Part print with two shaded views. Sizes in mm from the minimum x, y, z corner. Give positions to 0.01 mm unless a question says otherwise; leave off trailing zeros. Order: outer loops, then holes, each group sorted by start corner. A loop starts at its lowest first (then second) coordinate and runs counter-clockwise, first axis right, second up.
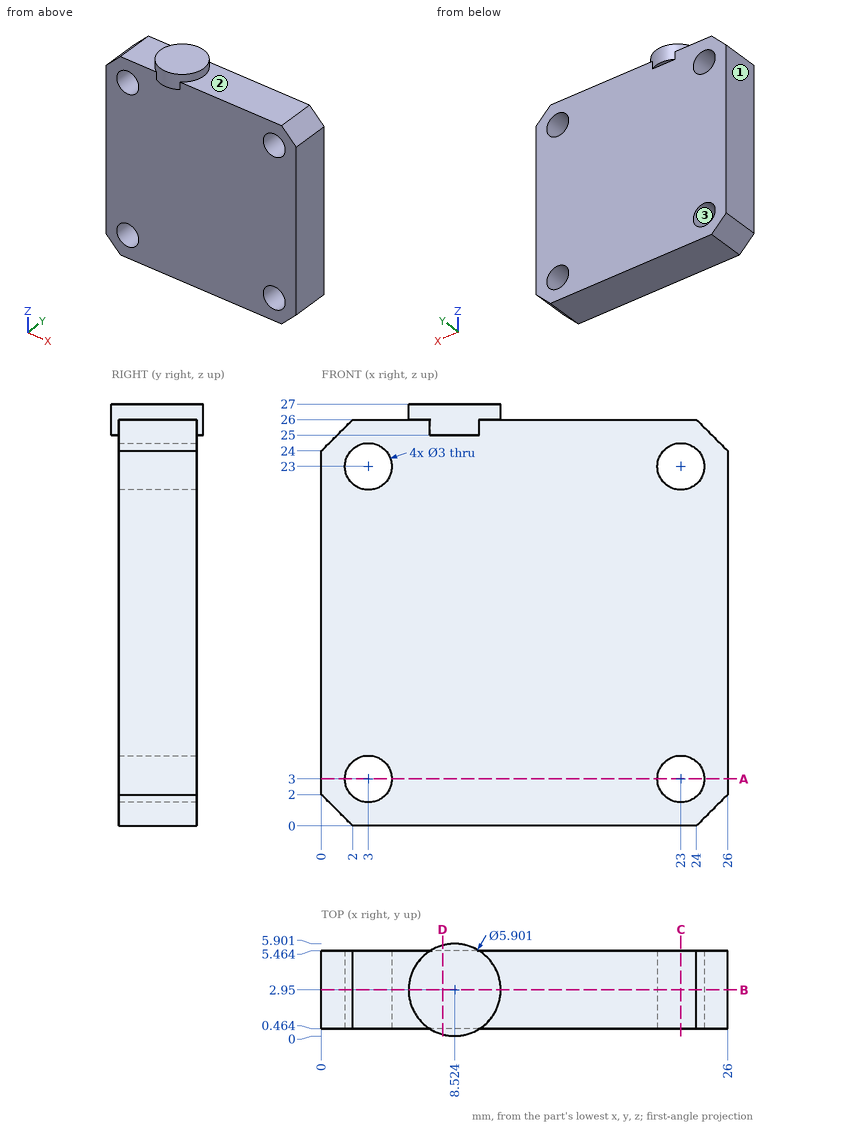
1. Saw through at D-D on x = 7.75. Give the cut face in (y, z), plus the area to 3 significant figures.
2. Saw through at C-C on x = 23. Give the cut face in (y, z).
3. Pin check, flat tips, straight feed: P1, Ø4, axis at x = 3, z = 23, coming from the +Y side; P2, Ø3.5, axis at x = 23, z = 3, coming from the -Y side. Stop position of each tip, or through.
4. Mould opens along Z. For the marked faces 1, 2 and 3 say: released by +Z, released by -Z, zero draft, split by the parting line, or undercut.
5. Saw through at A-A on z = 3. Give the cut face in (x, y).
6. Saw through at B-B on y = 2.95. Give the cut face in (x, z).
7. Wall check: line 1 (X direction, y = 2.4, z = 23); line 2 (X direction, y = 3.2, z = 2); line 3 (Z direction, x = 21.75, y = 4.5). Give the ranges that are in metal, low to high.
Reported:
1. outline: (0.1, 25) - (0.46, 25) - (0.46, 0) - (5.46, 0) - (5.46, 25) - (5.8, 25) - (5.8, 27) - (0.1, 27) - close
1. area: 136 mm2
2. outline: (0.46, 0) - (5.46, 0) - (5.46, 1.5) - (0.46, 1.5) - close; (0.46, 4.5) - (5.46, 4.5) - (5.46, 21.5) - (0.46, 21.5) - close; (0.46, 24.5) - (5.46, 24.5) - (5.46, 26) - (0.46, 26) - close
3. P1: stops at y = 5.46
3. P2: stops at y = 0.46
4. face 1: zero draft
4. face 2: released by +Z
4. face 3: undercut
5. outline: (0, 0.46) - (1.5, 0.46) - (1.5, 5.46) - (0, 5.46) - close; (4.5, 0.46) - (21.5, 0.46) - (21.5, 5.46) - (4.5, 5.46) - close; (24.5, 0.46) - (26, 0.46) - (26, 5.46) - (24.5, 5.46) - close
6. outline: (0, 2) - (2, 0) - (24, 0) - (26, 2) - (26, 24) - (24, 26) - (11.47, 26) - (11.47, 27) - (5.57, 27) - (5.57, 26) - (2, 26) - (0, 24) - close; hole circle Ø3 at (3, 3); hole circle Ø3 at (3, 23); hole circle Ø3 at (23, 3); hole circle Ø3 at (23, 23)
7. line 1: x = 0 to 1.5, 4.5 to 21.5, 24.5 to 26
7. line 2: x = 0 to 1.88, 4.12 to 21.88, 24.12 to 26
7. line 3: z = 0 to 2.17, 3.83 to 22.17, 23.83 to 26
